```python
from build123d import *

# Parameters (mm, degrees)
F0_W        = 76.2
F0_H        = 50.8
F1_DEPTH    = 6.35
F2_R        = 5.08
F3_T1_DEPTH = 93.0005208253
F3_T3_DEPTH = 67.6005208253


# Not quite as in the source:
# - a fillet or chamfer that OpenCascade refuses, or shapes differently, is made with other operations: its cross-section is extruded or revolved along the edge and cut away or added


with BuildPart() as f1:
    # F0 (on Top) → F1 (new body)
    with BuildSketch(Plane.XY):
        with Locations((38.1, -25.4)):
            Rectangle(F0_W, F0_H)
    extrude(amount=F1_DEPTH)

    # F2
    f2_edges = [f1.edges().sort_by_distance(p)[0] for p in [
        (38.1, 0, 6.35),
        (0, -25.4, 6.35),
        (38.1, -50.8, 6.35),
        (76.2, -25.4, 6.35),
    ]]
    fillet(f2_edges, radius=F2_R)

    # F3: fillet of radius 5.08 on 4 edges, made by hand

    # F3_s2 → F3_t1 (cut)
    with BuildSketch(Plane.YZ.offset(-8.4002604126)):
        with BuildLine():
            add(Edge.make_bspline(
                [(0, 1.27), (-1.4400446422, 0), (-3.3601041651, 0)],
                knots=[0, 0, 0, 1, 1, 1], degree=2, weights=[1, 1, 1]))
            Line((-3.3601041651, 0), (0, 0))
            Line((0, 0), (0, 1.27))
        make_face()
        with BuildLine():
            add(Edge.make_bspline(
                [(-47.4398958349, 0), (-49.3599553578, 0), (-50.8, 1.27)],
                knots=[0, 0, 0, 1, 1, 1], degree=2, weights=[1, 1, 1]))
            Line((-50.8, 1.27), (-50.8, 0))
            Line((-50.8, 0), (-47.4398958349, 0))
        make_face()
    extrude(amount=F3_T1_DEPTH, mode=Mode.SUBTRACT)

    # F3_s4 → F3_t3 (cut)
    with BuildSketch(Plane.XZ.offset(-8.4002604126)):
        with BuildLine():
            add(Edge.make_bspline(
                [(3.3601041651, 0), (1.4400446422, 0), (0, 1.27)],
                knots=[0, 0, 0, 1, 1, 1], degree=2, weights=[1, 1, 1]))
            Line((0, 1.27), (0, 0))
            Line((0, 0), (3.3601041651, 0))
        make_face()
        with BuildLine():
            add(Edge.make_bspline(
                [(76.2, 1.27), (74.7599553578, 0), (72.8398958349, 0)],
                knots=[0, 0, 0, 1, 1, 1], degree=2, weights=[1, 1, 1]))
            Line((72.8398958349, 0), (76.2, 0))
            Line((76.2, 0), (76.2, 1.27))
        make_face()
    extrude(amount=F3_T3_DEPTH, mode=Mode.SUBTRACT)


solid = f1.part
```
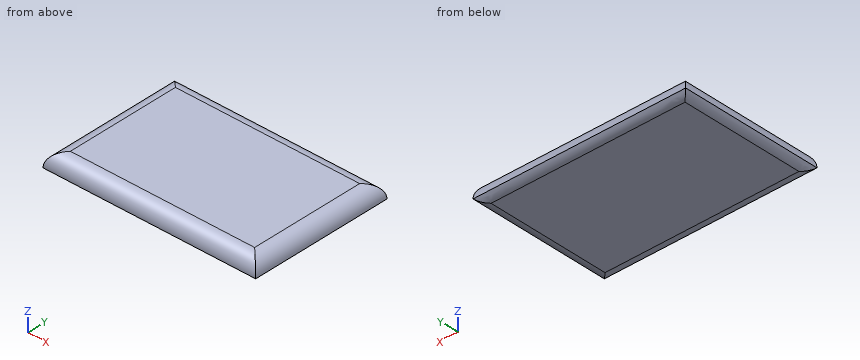
For this review, take the finished solid that the model builds, in its own axes (mm). Coordinates: 2 decimals unless noted, no trailing zeros. Order: outer loops, then holes, each group sorted by start corner. A loop starts at its lowest first (then second) coordinate and runs counter-clockwise, first axis right, second up. Notation, with made-up numbers: (72, 55.25) -> (125, 55.25) arc R14 ccw to (125, 79.25) -> close; hole circle Ø6 at (30, 4.5). An arc over 180 degrees is marked (long way). Answer as CSV lines item,"result".
Q1. Clearance check with a flat-ended pin moving along its axis: pin 1 Ø2 at (x, z) = (40, 4) entering from +Y. State where the tip first meets the part, or that it passes through.
Model answer:
pin 1,"stops at y = -0.3"
Q2. Wall thickness on line 1 along Z through (x, y) = (37, -46); line 2 along X through (y, z) = (-36.5, 3.25); line 3 along X through (y, z) = (-37, 2.5): over which ranges is each line inside the solid? List them lowest first. Write a range as [from, to].
Model answer:
line 1,"z = [0, 6.34]"
line 2,"x = [0.4, 75.8]"
line 3,"x = [0.15, 76.05]"
Q3. We need section A-A (z = 4.5). State the section outline as (x, y) points.
Model answer:
outline,"(1.16, -49.64) -> (75.04, -49.64) -> (75.04, -1.16) -> (1.16, -1.16) -> close"
